```python
from build123d import *

# Parameters (mm, degrees)
F0_R     = 56.205306
F1_DEPTH = 25


with BuildPart() as f1:
    # F0 (on Front) → F1 (new body)
    with BuildSketch(Plane.XZ):
        with BuildLine():
            Line((190, 100), (-190, 100))
            Line((-190, 100), (-570, 100))
            Line((-570, 100), (-570, 39.229718))
            ThreePointArc((-570, 39.229718), (-528.067085, -2.703197), (-570, -44.636112))
            Line((-570, -44.636112), (-570, -100))
            Line((-570, -100), (-190, -100))
            Line((-190, -100), (190, -100))
            ThreePointArc((190, -100), (290, 0), (190, 100))
        make_face()
        with Locations((190, 0)):
            Circle(F0_R, mode=Mode.SUBTRACT)
        with BuildLine():
            Line((-570, 39.229718), (-570, 100))
            ThreePointArc((-570, 100), (-625.122719, 83.435519), (-661.983853, 39.229718))
            Line((-661.983853, 39.229718), (-570, 39.229718))
        make_face()
        with BuildLine():
            Line((-570, -100), (-570, -44.636112))
            Line((-570, -44.636112), (-659.485292, -44.636112))
            ThreePointArc((-659.485292, -44.636112), (-622.613633, -85.040023), (-570, -100))
        make_face()
    extrude(amount=F1_DEPTH)


solid = f1.part
```
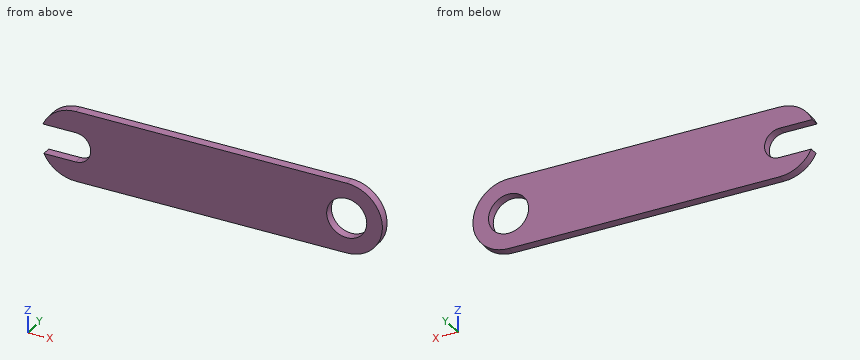
Read the model definition and answer for the solid it produces. Units are mm, in the model's axes. Coordinates: 2 decimals unless noted, no trailing zeros. Order: outer loops, then holes, each group sorted by start corner. A loop starts at its lowest first (then second) coordinate and runs counter-clockwise, first axis right, second up. Notation, with made-up numbers: (45.25, 22) - (61.25, 22) arc R5 cw to (61.25, 30) - close; hole circle Ø2 at (67.5, 38.25). An arc over 180 degrees is marked (long way). Answer as a JSON object with one key per item and string values. Group by question number.
Item 1: Section C-C (z = -35) is taken. Give the vertices of the cut face in (x, y), plus the area to 3 significant figures.
Item 2: Consider probe 1 along Z at (x, y) = (190, -15.75); probe 2 along Z at (x, y) = (-606.5, -10.75); probe 3 along X at (y, z) = (-18.75, 11.5). Determine where each line is inside the solid, lowest interval first. Write a range as from..to.
Item 3: Flat-ended cylindrical pins translate along their axes: P1, Ø10, axis at x = 20.5, z = -26, coming from the +Y side; P2, Ø12.5, axis at x = -601, y = -15.5, coming from the -Z side; P3, Ø2, axis at y = -16, z = 25.5, coming from the -X side; P4, Ø3, axis at y = -6, z = 60, coming from the +X side. Find the tip coordinate at first contact, or state that the pin passes through.
Item 4: Section B-B (y = -5.5) is taken. Give the vertices of the cut face in (x, z).
Item 5: Section A-A (x = -560.5) is taken. Give the vertices of the cut face in (y, z), plus the area to 3 significant figures.
Results are:
{
 "1": {"outline": "(-543.26, -25) - (146.02, -25) - (146.02, 0) - (-543.26, 0) - close; (233.98, -25) - (283.67, -25) - (283.67, 0) - (233.98, 0) - close", "area": "18,500 mm^2"},
 "2": {"probe 1": "z = -100..-56.21, 56.21..100", "probe 2": "z = -93.1..-44.64, 39.23..93.1", "probe 3": "x = -530.55..134.98, 245.02..289.34"},
 "3": {"P1": "stops at y = 0", "P2": "stops at z = -96.89", "P3": "stops at x = -539.91", "P4": "stops at x = 271.1"},
 "4": {"outline": "(-661.98, 39.23) - (-570, 39.23) arc R41.93 cw to (-570, -44.64) - (-659.49, -44.64) arc R100 ccw to (-570, -100) - (190, -100) arc R100 ccw to (190, 100) - (-570, 100) arc R100 ccw to start; hole circle Ø112.41 at (190, 0)"},
 "5": {"outline": "(-25, -100) - (0, -100) - (0, -43.55) - (-25, -43.55) - close; (-25, 38.14) - (0, 38.14) - (0, 100) - (-25, 100) - close", "area": "2,960 mm^2"}
}
